from build123d import *

# Parameters (mm, degrees)
SKETCH_1_R      = 1.3
SKETCH_1_R_2    = 1.1
EXTRUDE_1_DEPTH = 5
SKETCH_2_R      = 1.6
SKETCH_2_R_2    = 1.1
EXTRUDE_2_DEPTH = 4
EXTRUDE_START   = 4
SKETCH_3_R      = 1.1
SKETCH_3_R_2    = 1.3
EXTRUDE_3_DEPTH = 4
FILLET_1_R      = 5
FILLET_2_R      = 2.5


with BuildPart() as part:
    # ｽｹｯﾁ1 → ﾎﾞｽ - 押し出し1 (new body)
    with BuildSketch(Plane.XY):
        with BuildLine():
            Line((-8, 0), (8, 0))
            Line((8, 0), (8, 12))
            ThreePointArc((8, 12), (10, 18), (8, 24))
            Line((8, 24), (8, 36))
            Line((8, 36), (-8, 36))
            Line((-8, 36), (-8, 24))
            ThreePointArc((-8, 24), (-10, 18), (-8, 12))
            Line((-8, 12), (-8, 0))
        make_face()
        with Locations((0, 18)):
            Circle(SKETCH_1_R, mode=Mode.SUBTRACT)
        with Locations((0, 24)):
            Circle(SKETCH_1_R_2, mode=Mode.SUBTRACT)
        with Locations((4.242640687, 22.242640687)):
            Circle(SKETCH_1_R_2, mode=Mode.SUBTRACT)
        with Locations((6, 18)):
            Circle(SKETCH_1_R_2, mode=Mode.SUBTRACT)
        with Locations((4.242640687, 13.757359313)):
            Circle(SKETCH_1_R_2, mode=Mode.SUBTRACT)
        with Locations((0, 12)):
            Circle(SKETCH_1_R_2, mode=Mode.SUBTRACT)
        with Locations((-4.242640687, 13.757359313)):
            Circle(SKETCH_1_R_2, mode=Mode.SUBTRACT)
        with Locations((-6, 18)):
            Circle(SKETCH_1_R_2, mode=Mode.SUBTRACT)
        with Locations((-4.242640687, 22.242640687)):
            Circle(SKETCH_1_R_2, mode=Mode.SUBTRACT)
    extrude(amount=EXTRUDE_1_DEPTH)

    # ｽｹｯﾁ2 → ﾎﾞｽ - 押し出し2 (add)
    with BuildSketch(Plane.XZ):
        with BuildLine():
            Line((-8, 0), (8, 0))
            Line((8, 0), (8, 21))
            ThreePointArc((8, 21), (10, 27), (8, 33))
            Line((8, 33), (8, 37))
            Line((8, 37), (-8, 37))
            Line((-8, 37), (-8, 33))
            ThreePointArc((-8, 33), (-10, 27), (-8, 21))
            Line((-8, 21), (-8, 0))
        make_face()
        with Locations(Location((0, 27, 0), (0, 0, 270))):
            Circle(SKETCH_2_R, mode=Mode.SUBTRACT)
        with Locations(Location((6, 27, 0), (0, 0, 270))):
            Circle(SKETCH_2_R_2, mode=Mode.SUBTRACT)
        with Locations(Location((4.242640687, 22.757359313, 0), (0, 0, 270))):
            Circle(SKETCH_2_R_2, mode=Mode.SUBTRACT)
        with Locations(Location((0, 21, 0), (0, 0, 270))):
            Circle(SKETCH_2_R_2, mode=Mode.SUBTRACT)
        with Locations(Location((-4.242640687, 22.757359313, 0), (0, 0, 270))):
            Circle(SKETCH_2_R_2, mode=Mode.SUBTRACT)
        with Locations(Location((-6, 27, 0), (0, 0, 270))):
            Circle(SKETCH_2_R_2, mode=Mode.SUBTRACT)
        with Locations(Location((-4.242640687, 31.242640687, 0), (0, 0, 270))):
            Circle(SKETCH_2_R_2, mode=Mode.SUBTRACT)
        with Locations(Location((0, 33, 0), (0, 0, 270))):
            Circle(SKETCH_2_R_2, mode=Mode.SUBTRACT)
        with Locations(Location((4.242640687, 31.242640687, 0), (0, 0, 270))):
            Circle(SKETCH_2_R_2, mode=Mode.SUBTRACT)
    extrude(amount=EXTRUDE_2_DEPTH)

    # ｽｹｯﾁ3 → ﾎﾞｽ - 押し出し3 (add)
    with BuildSketch(Plane(origin=(0, 36, 0), x_dir=(1, 0, 0), z_dir=(0, 1, 0)).offset(EXTRUDE_START)):
        with BuildLine():
            Line((8, -5), (8, 0))
            Line((8, 0), (-8, 0))
            Line((-8, 0), (-8, -5))
            Line((-8, -5), (-8, -21))
            ThreePointArc((-8, -21), (-10, -27), (-8, -33))
            Line((-8, -33), (-8, -37))
            Line((-8, -37), (8, -37))
            Line((8, -37), (8, -33))
            ThreePointArc((8, -33), (10, -27), (8, -21))
            Line((8, -21), (8, -5))
        make_face()
        with Locations(Location((4.242640687, -22.757359313, 0), (0, 0, 90))):
            Circle(SKETCH_3_R, mode=Mode.SUBTRACT)
        with Locations(Location((0, -21, 0), (0, 0, 90))):
            Circle(SKETCH_3_R, mode=Mode.SUBTRACT)
        with Locations(Location((-4.242640687, -22.757359313, 0), (0, 0, 90))):
            Circle(SKETCH_3_R, mode=Mode.SUBTRACT)
        with Locations(Location((-6, -27, 0), (0, 0, 90))):
            Circle(SKETCH_3_R, mode=Mode.SUBTRACT)
        with Locations(Location((-4.242640687, -31.242640687, 0), (0, 0, 90))):
            Circle(SKETCH_3_R, mode=Mode.SUBTRACT)
        with Locations(Location((0, -33, 0), (0, 0, 90))):
            Circle(SKETCH_3_R, mode=Mode.SUBTRACT)
        with Locations(Location((4.242640687, -31.242640687, 0), (0, 0, 90))):
            Circle(SKETCH_3_R, mode=Mode.SUBTRACT)
        with Locations(Location((6, -27, 0), (0, 0, 90))):
            Circle(SKETCH_3_R, mode=Mode.SUBTRACT)
        with Locations(Location((0, -27, 0), (0, 0, 270))):
            Circle(SKETCH_3_R_2, mode=Mode.SUBTRACT)
    extrude(amount=-EXTRUDE_3_DEPTH)

    # ﾌｨﾚｯﾄ1
    fillet_1_edges = [part.edges().sort_by_distance(p)[0] for p in [
        (0, 36, 5),
        (0, -4, 0),
        (0, 0, 5),
        (0, 40, 0),
    ]]
    fillet(fillet_1_edges, radius=FILLET_1_R)

    # ﾌｨﾚｯﾄ2
    fillet_2_edges = [part.edges().sort_by_distance(p)[0] for p in [
        (8, 38, 21),
        (-8, 38, 21),
        (-8, 38, 33),
        (-8, 38, 37),
        (8, 38, 37),
        (8, 38, 33),
        (-8, 12, 2.5),
        (-8, 24, 2.5),
        (8, 24, 2.5),
        (8, 12, 2.5),
        (-8, -2, 21),
        (8, -2, 21),
        (8, -2, 33),
        (8, -2, 37),
        (-8, -2, 37),
        (-8, -2, 33),
    ]]
    fillet(fillet_2_edges, radius=FILLET_2_R)


solid = part.part
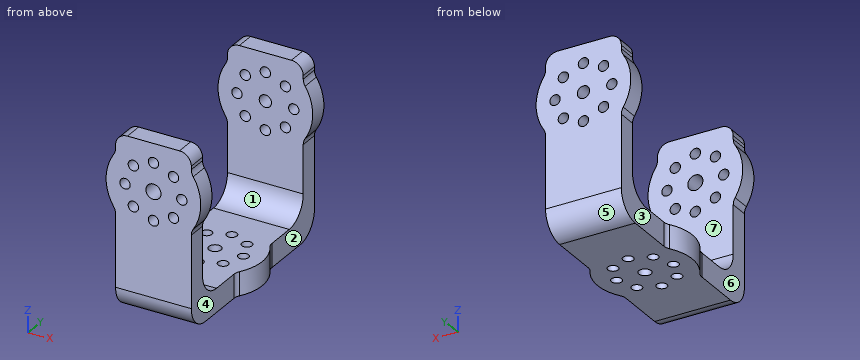
The model under review builds one solid part; all positions refer to its coordinate system, in mm. Face numbers are marked on the shaded views. A direction names the side the tool comes from. Coordinates: 2 decimals unless noted, no trailing zeros. Loops run counter-clockwise (first coordinate to the right, second up) from the corner with the lowest first, then second, coordinate; pieces in that order, holes last. Notation, with made-up numbers: (5, 39.5) -> (18, 39.5) arc R20 ccw to (18, 73.5) -> close; hole circle Ø8 at (44.25, 13.5). An arc over 180 degrees is marked (long way). Use a Markdown table: item, result. Add a question column.
1. Add section D-D on z = 31. Write out the cut boundary in (x, y), plus the area to 3 significant figures.
2. Draft analysis for pull direction Y (two halves, no side actions). For the marked faces 5, 6 and 7, state which applies: pulls with the +Y half, pulls with the -Y half, needs draft (parallel to the pull), parting line crosses it, or undercut.
3. Add section B-B on z = 27. Give the number of separate pieces and of enclosed holes in the cut face, plus the area to 3 significant figures.
4. Clearance check with flat-ended pins moving along their axes: pin 1 Ø0.6 at (y, z) = (-2.5, 34) entering from +X; pin 2 Ø1.5 at (y, z) = (25, 4) entering from -X; pin 3 Ø3 at (x, y) = (0, 18) entering from +Z. State where each tip first meets the part, or that it passes through.
5. Add section A-A on z = 11. Write out the cut boundary in (x, y).
6. Machinability: for the marked faces 1, 2, 3 and 4, which of the approach directions +Z, -Z, +X, -X, +Y, -Y give a long, thin tool a straight path to every point of the face, cutting with its end or side? Answer none if there is none.
7. To check wall thickness, follow line 1 (X direction, y = 38, z = 27); line 2 (X direction, y = -2.3, z = 27); line 3 (Y direction, x = 6, z = 21). State the ranges of each line that lie inside material, in increasing order.
8. Add section C-C on x = 6.5. Write out the cut boundary in (y, z).
Returned:
| question | item | result |
|---|---|---|
| 1 | outline | (-9.17, -4) -> (-5.32, -4) -> (-5.32, 0) -> (-9.17, 0) -> close; (-9.17, 36) -> (-5.32, 36) -> (-5.32, 40) -> (-9.17, 40) -> close; (-3.17, -4) -> (3.17, -4) -> (3.17, 0) -> (-3.17, 0) -> close; (-3.17, 36) -> (3.17, 36) -> (3.17, 40) -> (-3.17, 40) -> close; (5.32, -4) -> (9.17, -4) -> (9.17, 0) -> (5.32, 0) -> close; (5.32, 36) -> (9.17, 36) -> (9.17, 40) -> (5.32, 40) -> close |
| 1 | area | 112 mm² |
| 2 | face 5 | pulls with the +Y half |
| 2 | face 6 | needs draft |
| 2 | face 7 | undercut |
| 3 | separate pieces | 8 |
| 3 | enclosed holes | 0 |
| 3 | area | 102 mm² |
| 4 | pin 1 | stops at x = 8 |
| 4 | pin 2 | stops at x = -8.06 |
| 4 | pin 3 | stops at z = 5 |
| 5 | outline | (-8, -4) -> (8, -4) -> (8, 0) -> (-8, 0) -> close; (-8, 36) -> (8, 36) -> (8, 40) -> (-8, 40) -> close |
| 6 | face 1 | +Z, +X, -X |
| 6 | face 2 | -Z, +X, +Y |
| 6 | face 3 | -Z, -X, +Y |
| 6 | face 4 | -Z, +X, -Y |
| 7 | line 1 | x = -10 to -7.1, -4.9 to -1.3, 1.3 to 4.9, 7.1 to 10 |
| 7 | line 2 | x = -10 to -7.1, -4.9 to -1.6, 1.6 to 4.9, 7.1 to 10 |
| 7 | line 3 | y = -4 to 0, 36 to 40 |
| 8 | outline | (-4, 5) arc R5 ccw to (1, 0) -> (17.02, 0) -> (17.02, 5) -> (5, 5) arc R5 cw to (0, 10) -> (0, 26.02) -> (-4, 26.02) -> close; (-4, 27.98) -> (0, 27.98) -> (0, 36.79) -> (-4, 36.79) -> close; (18.98, 0) -> (35, 0) arc R5 ccw to (40, 5) -> (40, 26.02) -> (36, 26.02) -> (36, 10) arc R5 cw to (31, 5) -> (18.98, 5) -> close; (36, 27.98) -> (40, 27.98) -> (40, 36.79) -> (36, 36.79) -> close |
